```python
from build123d import *

# Parameters (mm, degrees)
F1_DEPTH = 25.4
F2_R     = 1.26999


# Not quite as in the source:
# - a fillet or chamfer is up to 0.001 mm smaller than in the source, because OpenCascade refuses the exact size


with BuildPart() as f1:
    # F0 (on Right) → F1 (new body)
    with BuildSketch(Plane.YZ):
        Polygon((14.605, 1.27), (-0.635, 1.27), (-7.9526191413, 6.35), (-10.4926191413, 6.35), (-10.4926191413, 3.81), (-7.9526191413, 3.81), (-5.715, 1.27), (-5.715, -1.27), (14.605, -1.27), align=None)
    extrude(amount=F1_DEPTH)

    # F2 (radius 1.27 in the source; OpenCascade refuses exactly that, so slightly less here)
    f2_edges = [f1.edges().sort_by_distance(p)[0] for p in [
        (12.7, -10.492619, 6.35),
        (12.7, -7.952619, 6.35),
        (12.7, -10.492619, 3.81),
        (12.7, 14.605, 1.27),
        (12.7, 14.605, -1.27),
        (12.7, -5.715, -1.27),
        (25.4, 6.985, 1.27),
        (0, 6.985, 1.27),
        (25.4, 4.445, -1.27),
        (0, 4.445, -1.27),
    ]]
    fillet(f2_edges, radius=F2_R)


solid = f1.part
```
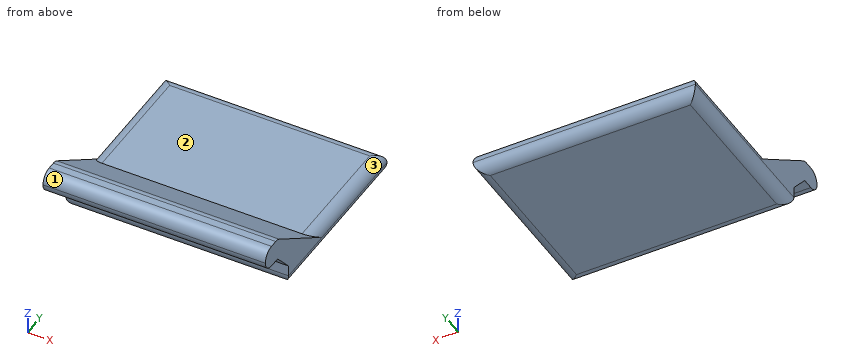
Verification items for the finished model (mm, model axes). Face numbers are marked on the shaded views. A direction names the side the tool comes from. Give positions to 0.01 mm unless a question says otherwise; leave off trailing zeros. Order: outer loops, then holes, each group sorted by start corner. A loop starts at its lowest first (then second) coordinate and runs counter-clockwise, first axis right, second up. Notation, with made-up numbers: M -20,-9.5 L 18,-9.5 A15 cw 18,-0.5 Z; hole C 59.5,50.25 d4. An arc over 180 degrees is marked long. Return JSON: item names as keys, results as strings. Group by question number.
1) Scan lines: line 1 (Z direction, x = 17.5, y = -9); line 2 (Z direction, x = 9.75, y = 6); line 3 (Y direction, x = 10.25, z = 1.5). Record each from-to range of solid material in increasing order.
2) Section check D-D on y = -0.25. Record the cut outline in (x, z).
3) Section check C-C on z = 0.5. Record the cut outline in (x, y) (3 decimals).
4) Go/stop test with flat-tipped pins: pin 1 Ø4 at (x, y) = (21.5, -3.5) entering from +Z; pin 2 Ø4 at (y, z) = (10, 1) entering from -X; pin 3 Ø1 at (x, z) = (13, 0.5) entering from -Y (3 decimals); pin 4 Ø4 at (x, y) = (15, 9.5) entering from +Z. Record where each tip stops, or that it passes through.
5) Access from +Z, -Z, +X, -X, +Y, -Y to the whole of each face (thin tool, end or side, straight path). Record for the marked faces 1, 2 and 3.
Answer block:
{
 "1": {"line 1": "z = 3.81 to 6.35", "line 2": "z = -1.27 to 1.27", "line 3": "y = -5.92 to -0.97"},
 "2": {"outline": "M 0,0 A1.27 ccw 1.27,-1.27 L 24.13,-1.27 A1.27 ccw 25.4,0 L 25.4,1 L 24.91,1 A1.27 ccw 24.13,1.27 L 1.27,1.27 A1.27 ccw 0.49,1 L 0,1 Z"},
 "3": {"outline": "M 0,-5.715 L 25.4,-5.715 L 25.4,0.474 L 25.297,0.474 L 25.297,14.502 L 0.103,14.502 L 0.103,0.474 L 0,0.474 Z"},
 "4": {"pin 1": "stops at z = 4.65", "pin 2": "stops at x = 0", "pin 3": "stops at y = -5.715", "pin 4": "stops at z = 1.27"},
 "5": {"face 1": "+Z, +X, -X, -Y", "face 2": "+Z, +X, -X, +Y", "face 3": "+Z, +X, +Y"}
}
